Verification items for the finished model (mm, model axes). A direction names the side the tool comes from. Coordinates: 2 decimals unless noted, no trailing zeros. Loops run counter-clockwise (first coordinate to the right, second up) from the corner with the lowest first, then second, coordinate; pieces in that order, holes last. Notation, with made-up numbers: (18.25, 76) - (27.25, 76) arc R37 ccw to (27.25, 115) - close; hole circle Ø5 at (21, 53). An arc over 180 degrees is marked (long way). One line per item, written item: value. Start each with the question number.
(1) Section check D-D (z = 88). Record the boundary of the cut face in (x, y), plus the area to 3 significant figures.
(2) Gauge pin test, flat ends, axial feed: P1, Ø15.5, axis at x = -2.5, z = 15, coming from the +Y side; P2, Ø8, axis at y = -21.5, z = 14, coming from the -X side; P3, Ø3, axis at y = -30, z = 43.5, coming from the -X side; P4, Ø10, axis at y = 22.5, z = 49, coming from the -X side. Record the tip position at first contact, or that the pin passes through.
(3) Set-up check for faces 1 (the face through (10, -5, 69.777)), 2 (the face through (22, -33, 40)), 3 (the face through (2, -17.5, 47)): record each of +Z, -Z, +X, -X, +Y, -Y from which the full face is reachable in a straight line by a thin tool's end or side.
(4) Thickness scan on probe 1 along Z at (x, y) = (47, -32); probe 2 along Z at (x, y) = (30.5, -28); probe 3 along X at (y, z) = (-28.5, 122.5). Record the ranges inside material, lowest first. Write a range as [from, to].
(5) Section check B-B (z = 15). Record the boundary of the cut face in (x, y).
(6) Section check A-A (y = -30.5). Record the boundary of the cut face in (x, z).
(7) Draft check along Z on faces 4 (the face through (47.764, -32.43, 114.006)), 5 (the face through (10, -5, 63.777)), 6 (the face through (3.471, 4.685, 66.819)). Enter one of: +Z half, -Z half, draft (parallel to the pull), parting line (faces both ways), or undercut.
(8) Section check C-C (x = 40). Record the boundary of the cut face in (y, z), plus the area to 3 significant figures.
```python
from build123d import *

# Parameters (mm, degrees)
SKETCH2_R                = 10
BOSS_EXTRUDE1_DEPTH      = 135
SKETCH4_W                = 90
SKETCH4_H                = 10
CUT_EXTRUDE1_DEPTH       = 30
SKETCH6_W                = 90
SKETCH6_H                = 10
CUT_EXTRUDE2_DEPTH       = 30
CUT_EXTRUDE3_DEPTH       = 30
CUT_EXTRUDE4_START       = -30
CUT_EXTRUDE4_DEPTH       = 30
SKETCH11_W               = 55
SKETCH11_H               = 20
CUT_EXTRUDE5_DEPTH       = 167.527024834
SKETCH12_R               = 6
CUT_EXTRUDE6_DEPTH       = 165.335784295
SKETCH13_R               = 6
CUT_EXTRUDE7_DEPTH       = 165.335784295
SKETCH14_W               = 6
SKETCH14_H               = 30
BOSS_EXTRUDE3_DEPTH      = 10
SKETCH15_W               = 6
SKETCH15_H               = 30
BOSS_EXTRUDE4_DEPTH      = 10
CUT_EXTRUDE8_DEPTH       = 149.105536696
CUT_EXTRUDE8_DEPTH_BACK  = 149.105536696
CUT_EXTRUDE9_DEPTH       = 149.105536696
CUT_EXTRUDE9_DEPTH_BACK  = 149.105536696
BOSS_EXTRUDE5_DEPTH      = 50
BOSS_EXTRUDE5_DEPTH_BACK = 10
SKETCH18_W               = 6
SKETCH18_H               = 45
CUT_EXTRUDE10_DEPTH      = 106.048466338
CUT_EXTRUDE10_DEPTH_BACK = 106.048466338


with BuildPart() as part:
    # Sketch2 → Boss-Extrude1 (new body)
    with BuildSketch(Plane.XY):
        with BuildLine():
            Line((67.5, 17.5), (67.5, -37.5))
            Line((67.5, -37.5), (-22.5, -37.5))
            Line((-22.5, -37.5), (-22.5, -17.5))
            Line((-22.5, -17.5), (27.5, -17.5))
            Line((27.5, -17.5), (27.5, 17.5))
            ThreePointArc((27.5, 17.5), (47.5, 37.5), (67.5, 17.5))
        make_face()
        with Locations((47.5, 17.5)):
            Circle(SKETCH2_R, mode=Mode.SUBTRACT)
    extrude(amount=BOSS_EXTRUDE1_DEPTH)

    # Sketch4 → Cut-Extrude1 (cut)
    with BuildSketch(Plane.XY.offset(135)):
        with Locations((22.5, -22.5)):
            Rectangle(SKETCH4_W, SKETCH4_H)
    extrude(amount=-CUT_EXTRUDE1_DEPTH, mode=Mode.SUBTRACT)

    # Sketch6 → Cut-Extrude2 (cut)
    with BuildSketch(Plane(origin=(0, 0, 0), x_dir=(-1, 0, 0), z_dir=(0, 0, -1))):
        with Locations((-22.5, -22.5)):
            Rectangle(SKETCH6_W, SKETCH6_H)
    extrude(amount=-CUT_EXTRUDE2_DEPTH, mode=Mode.SUBTRACT)

    # Sketch9 → Cut-Extrude3 (cut)
    with BuildSketch(Plane(origin=(0, 0, 0), x_dir=(-1, 0, 0), z_dir=(0, 0, -1))):
        with BuildLine():
            Line((-67.5, -17.5), (-67.5, 17.5))
            ThreePointArc((-67.5, 17.5), (-47.5, 37.5), (-27.5, 17.5))
            Line((-27.5, 17.5), (-27.5, -17.5))
            Line((-27.5, -17.5), (-67.5, -17.5))
        make_face()
    extrude(amount=-CUT_EXTRUDE3_DEPTH, mode=Mode.SUBTRACT)

    # Sketch10 → Cut-Extrude4 (cut)
    with BuildSketch(Plane.XY.offset(135).offset(CUT_EXTRUDE4_START)):
        with BuildLine():
            Line((27.5, -17.5), (67.5, -17.5))
            Line((67.5, -17.5), (67.5, 17.5))
            ThreePointArc((67.5, 17.5), (47.5, 37.5), (27.5, 17.5))
            Line((27.5, 17.5), (27.5, -17.5))
        make_face()
    extrude(amount=CUT_EXTRUDE4_DEPTH, mode=Mode.SUBTRACT)

    # Sketch11 → Cut-Extrude5 (cut, through all)
    with BuildSketch(Plane.ZY.offset(22.5)):
        with Locations((67.5, -37.5)):
            Rectangle(SKETCH11_W, SKETCH11_H)
    extrude(amount=-CUT_EXTRUDE5_DEPTH, mode=Mode.SUBTRACT)

    # Sketch12 → Cut-Extrude6 (cut, through all)
    with BuildSketch(Plane(origin=(0, -27.5, 0), x_dir=(1, 0, 0), z_dir=(0, 1, 0))):
        with Locations(Location((-2.5, -120, 0), (0, 0, 270))):
            Circle(SKETCH12_R)
        with Locations(Location((47.5, -120, 0), (0, 0, 270))):
            Circle(SKETCH12_R)
    extrude(amount=-CUT_EXTRUDE6_DEPTH, mode=Mode.SUBTRACT)

    # Sketch13 → Cut-Extrude7 (cut, through all)
    with BuildSketch(Plane(origin=(0, -27.5, 0), x_dir=(1, 0, 0), z_dir=(0, 1, 0))):
        with Locations(Location((47.5, -15, 0), (0, 0, 180))):
            Circle(SKETCH13_R)
        with Locations(Location((-2.5, -15, 0), (0, 0, 180))):
            Circle(SKETCH13_R)
    extrude(amount=-CUT_EXTRUDE7_DEPTH, mode=Mode.SUBTRACT)

    # Sketch14 → Boss-Extrude3 (add)
    with BuildSketch(Plane(origin=(0, -27.5, 0), x_dir=(1, 0, 0), z_dir=(0, 1, 0))):
        with Locations((22.5, -120)):
            Rectangle(SKETCH14_W, SKETCH14_H)
    extrude(amount=BOSS_EXTRUDE3_DEPTH)

    # Sketch15 → Boss-Extrude4 (add)
    with BuildSketch(Plane(origin=(0, -27.5, 0), x_dir=(1, 0, 0), z_dir=(0, 1, 0))):
        with Locations((22.5, -15)):
            Rectangle(SKETCH15_W, SKETCH15_H)
    extrude(amount=BOSS_EXTRUDE4_DEPTH)

    # Sketch16 → Cut-Extrude8 (cut, two sides: drawn at the far end of the back side and taken through both)
    with BuildSketch(Plane.ZY.offset(-19.5).offset(-CUT_EXTRUDE8_DEPTH_BACK)):
        Polygon((105, -17.5), (135, -27.5), (135, -17.5), align=None)
    extrude(amount=CUT_EXTRUDE8_DEPTH + CUT_EXTRUDE8_DEPTH_BACK, mode=Mode.SUBTRACT)

    # Sketch17 → Cut-Extrude9 (cut, two sides: drawn at the far end of the back side and taken through both)
    with BuildSketch(Plane.ZY.offset(-19.5).offset(-CUT_EXTRUDE9_DEPTH_BACK)):
        Polygon((30, -17.5), (0, -27.5), (0, -17.5), align=None)
    extrude(amount=CUT_EXTRUDE9_DEPTH + CUT_EXTRUDE9_DEPTH_BACK, mode=Mode.SUBTRACT)

    # Sketch18 → Boss-Extrude5 (add, two sides: drawn at the far end of the back side and taken through both)
    with BuildSketch(Plane.ZY.offset(-27.5).offset(-BOSS_EXTRUDE5_DEPTH_BACK)):
        with Locations((66.77724886, 5)):
            Rectangle(SKETCH18_W, SKETCH18_H)
    extrude(amount=BOSS_EXTRUDE5_DEPTH + BOSS_EXTRUDE5_DEPTH_BACK)

    # Sketch19 → Cut-Extrude10 (cut, two sides: drawn at the far end of the back side and taken through both)
    with BuildSketch(Plane(origin=(0, 0, 63.77724886), x_dir=(-1, 0, 0), z_dir=(0, 0, -1)).offset(-CUT_EXTRUDE10_DEPTH_BACK)):
        Polygon((22.5, -17.5), (-30.179491924, 27.5), (22.5, 27.5), align=None)
    extrude(amount=CUT_EXTRUDE10_DEPTH + CUT_EXTRUDE10_DEPTH_BACK, mode=Mode.SUBTRACT)


solid = part.part
```
Responses:
1. outline: (-22.5, -27.5) - (67.5, -27.5) - (67.5, 17.5) arc R20 ccw to (27.5, 17.5) - (27.5, -17.5) - (-22.5, -17.5) - close; hole circle Ø20 at (47.5, 17.5)
1. area: 2,610 mm²
2. P1: stops at y = -27.5
2. P2: stops at x = 19.5
2. P3: passes through
2. P4: stops at x = 27.5
3. face 1: +Z, -X, +Y
3. face 2: +X, -X, -Y
3. face 3: -Z, -X, +Y
4. probe 1: z = [0, 9.02], [20.98, 40], [95, 114.02], [125.98, 135]
4. probe 2: z = [0, 40], [95, 135]
4. probe 3: x = [-22.5, -7.95], [2.95, 42.05], [52.95, 67.5]
5. outline: (-22.5, -37.5) - (-8.5, -37.5) - (-8.5, -27.5) - (-22.5, -27.5) - close; (3.5, -37.5) - (41.5, -37.5) - (41.5, -27.5) - (25.5, -27.5) - (25.5, -22.5) - (19.5, -22.5) - (19.5, -27.5) - (3.5, -27.5) - close; (53.5, -37.5) - (67.5, -37.5) - (67.5, -27.5) - (53.5, -27.5) - close
6. outline: (-22.5, 0) - (67.5, 0) - (67.5, 40) - (-22.5, 40) - close; (-22.5, 95) - (67.5, 95) - (67.5, 135) - (-22.5, 135) - close; hole circle Ø12 at (-2.5, 15); hole circle Ø12 at (-2.5, 120); hole circle Ø12 at (47.5, 15); hole circle Ø12 at (47.5, 120)
7. face 4: undercut
7. face 5: -Z half
7. face 6: draft
8. outline: (-37.5, 0) - (-27.5, 0) - (-27.5, 30) - (10.89, 30) - (10.89, 105) - (-27.5, 105) - (-27.5, 135) - (-37.5, 135) - (-37.5, 95) - (-27.5, 95) - (-27.5, 40) - (-37.5, 40) - close; (24.11, 30) - (36.04, 30) - (36.04, 105) - (24.11, 105) - close
8. area: 4,570 mm²
